Read the model definition and answer for the solid it produces. Units are mm, in the model's axes. A direction names the side the tool comes from. Coordinates: 2 decimals unless noted, no trailing zeros. Loops run counter-clockwise (first coordinate to the right, second up) from the corner with the lowest first, then second, coordinate; pieces in that order, holes last. Notation, with made-up numbers: (-39.5, 12) - (-11.5, 12) arc R30 cw to (-11.5, 47) - close; hole circle Ø4 at (0, 67.5). An arc over 180 degrees is marked (long way). Use one line per item in the form item = value. Start each with the question number.
1) Consider line 1 (Y direction, x = 145, z = 0); line 2 (X direction, y = -91, z = 51); line 3 (Z direction, x = 14, y = 151). Determine where each line is inside the solid, lowest interval first.
2) A cutting plane is placed at A-A (z = 0). Give the vertices of the cut face in (x, y).
3) Which of the six approach directions +Z, -Z, +X, -X, +Y, -Y give full straight-line access (tool end or side, diameter ignored) to faces 1 (the face through (140, 2, 2)), 2 (the face through (74, 175, 2))?
4) The mould has two halves that part along Z. Classify faces 3 (the face through (145.07, -156.195, 34.685)), 4 (the face through (76.05, 165.979, 166.445)), 5 (the face through (76.05, -166.445, -165.979)): released by +Z, released by -Z, zero draft, split by the parting line, or undercut.
5) This flat-tipped pin is pushed along its axis until it touches: P1, Ø4, axis at y = 93, z = 26, coming from the +X side. Where does it stop, or does it pass through?
from build123d import *

# Parameters (mm, degrees)
IZIM1_W                     = 350
IZIM1_H                     = 350
Y_KSEKLIK_EKSTR_ZYON1_DEPTH = 150
IZIM2_R                     = 160
KES_EKSTR_ZYON1_DEPTH       = 10
RADYUS1_R                   = 30


with BuildPart() as part:
    # Çizim1 → Yükseklik-Ekstrüzyon1 (new body)
    with BuildSketch(Plane(origin=(0, 0, 0), x_dir=(0, 0, -1), z_dir=(1, 0, 0))):
        Rectangle(IZIM1_W, IZIM1_H)
    extrude(amount=Y_KSEKLIK_EKSTR_ZYON1_DEPTH)

    # Çizim2 → Kes-Ekstrüzyon1 (cut)
    with BuildSketch(Plane(origin=(150, 0, 0), x_dir=(0, 0, -1), z_dir=(1, 0, 0))):
        Circle(IZIM2_R)
    extrude(amount=-KES_EKSTR_ZYON1_DEPTH, mode=Mode.SUBTRACT)

    # Radyus1
    radyus1_edges = [part.edges().sort_by_distance(p)[0] for p in [
        (75, -175, -175),
        (75, -175, 175),
        (75, 175, 175),
        (75, 175, -175),
    ]]
    fillet(radyus1_edges, radius=RADYUS1_R)


solid = part.part
Found:
q1.line_1 = -175 to -160, 160 to 175
q1.line_2 = 0 to 140
q1.line_3 = -174.39 to 174.39
q2.outline = (0, -175) - (150, -175) - (150, -160) - (140, -160) - (140, 160) - (150, 160) - (150, 175) - (0, 175) - close
q3.face_1 = +X
q3.face_2 = +Z, -Z, +X, -X, +Y
q4.face_3 = undercut
q4.face_4 = released by +Z
q4.face_5 = released by -Z
q5.P1 = 140
